The figure shows three views and two pictorial views of one solid part (mm, origin at its lowest corner). Answer the questions. A direction names the side the tool comes from. Give positions to 0.01 mm unless a question says otherwise; leave off trailing zeros. Write each loop counter-clockwise with the first axis right and the second up, starting at its lowest first coordinate (ties: lowest second). Pieces come first, ordered by that corner, then holes. Notation, with made-up numbers: (40.5, -39.5) - (59.5, -39.5) arc R27 cw to (59.5, -21.5) - close; hole circle Ø2 at (39.25, -25). An arc over 180 degrees is marked (long way). One line per question, with ' | ' between items. Start each with the question number.
1. The mould has two halves that part along X. Classify the marked faces 3, 4 and 5: +X half, -X half, draft (parallel to the pull), parting line (faces both ways), or undercut.
2. A cutting plane is placed at D-D (y = 5). Determine the outline of the cut face in (x, z).
3. Given P1, Ø1.5, axis at x = 21.5, z = 8.5, coming from the -Y side; P2, Ø10, axis at x = 8.5, y = 10, coming from the +Z side; P3, Ø12, axis at x = 22, z = 23, coming from the -Y side, each flat-ended and moving along its own axis, determine where each tip first touches the part or whether it passes through.
4. A cutting plane is placed at C-C (x = 57). Determine the outline of the cut face in (y, z) (3 decimals), then the cut area to 3 significant figures.
5. Find the intervals of material crossed by L1, parallel to X at y = 4, z = 16.5; L2, parallel to Z at x = 24, y = 16.51 (3 decimals), in increasing order. Write a range as from..to.
6. For the marked faces 1 and 2, determine the directions among +Z, -Z, +X, -X, +Y, -Y from which every point of the face is accessible in a straight line to the end or side of a thin tool.
7. A cutting plane is placed at A-A (y = 16.51). Determine the outline of the cut face in (x, z) (3 decimals), then the cut area to 3 significant figures.
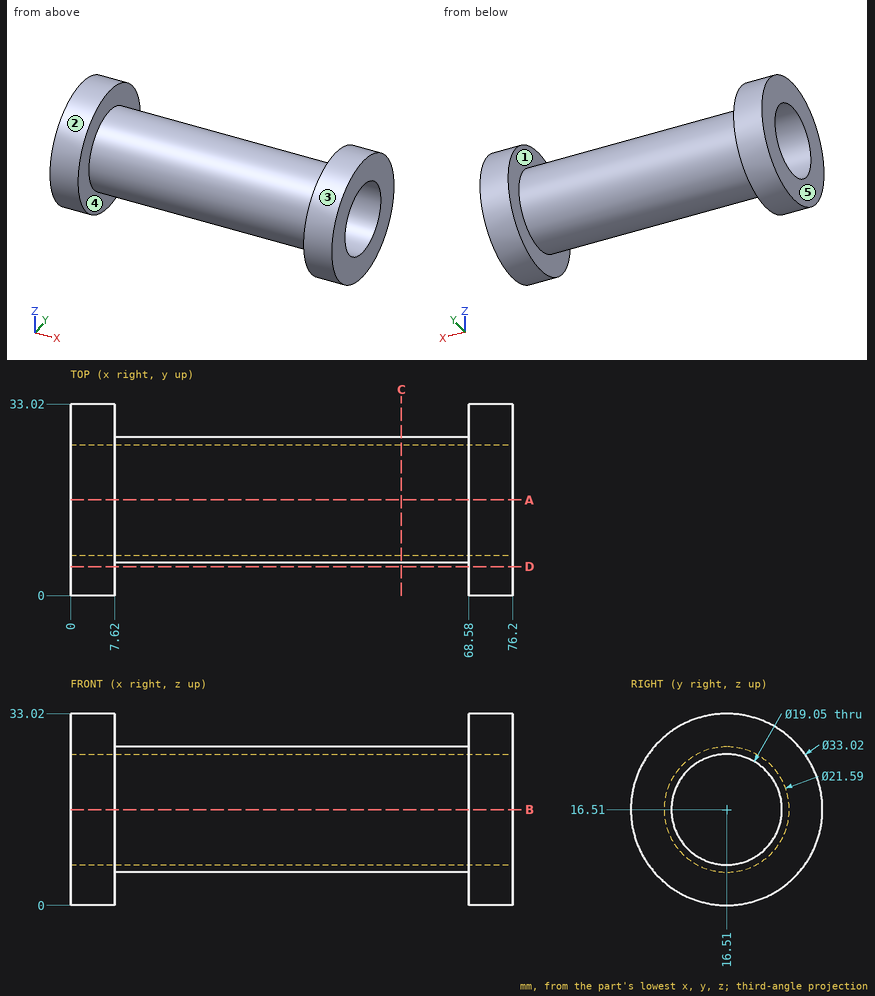
Determined:
1) face 3: draft | face 4: undercut | face 5: -X half
2) outline: (0, 4.67) - (7.62, 4.67) - (7.62, 28.35) - (0, 28.35) - close; (68.58, 4.67) - (76.2, 4.67) - (76.2, 28.35) - (68.58, 28.35) - close
3) P1: y = 8.52 | P2: z = 32.94 | P3: y = 5.73
4) outline: circle Ø21.59 at (16.51, 16.51); hole circle Ø19.05 at (16.51, 16.51) | area: 81.1 mm2
5) L1: 0..7.62, 68.58..76.2 | L2: 5.715..6.985, 26.035..27.305
6) face 1: none | face 2: +X, -X
7) outline: (0, 0) - (7.62, 0) - (7.62, 5.715) - (68.58, 5.715) - (68.58, 0) - (76.2, 0) - (76.2, 6.985) - (0, 6.985) - close; (0, 26.035) - (76.2, 26.035) - (76.2, 33.02) - (68.58, 33.02) - (68.58, 27.305) - (7.62, 27.305) - (7.62, 33.02) - (0, 33.02) - close | area: 368 mm2
